Input: part model. Units: mm. Frame: model coordinates. Face numbers are marked on the shaded views. A direction names the side the tool comes from. Give positions to 0.01 mm unless a question says otherwise; leave off trailing zeros. Order: outer loops, then holes, each group sorted by start corner. A loop starts at its lowest first (then second) coordinate and runs counter-clockwise, first axis right, second up. Notation, with made-up numbers: (72, 50.25) - (95, 50.25) arc R11 cw to (95, 68.25) - close; hole circle Ø8 at (-32.75, 61.5). An arc over 180 degrees is marked (long way). Use a Markdown table: item, result.
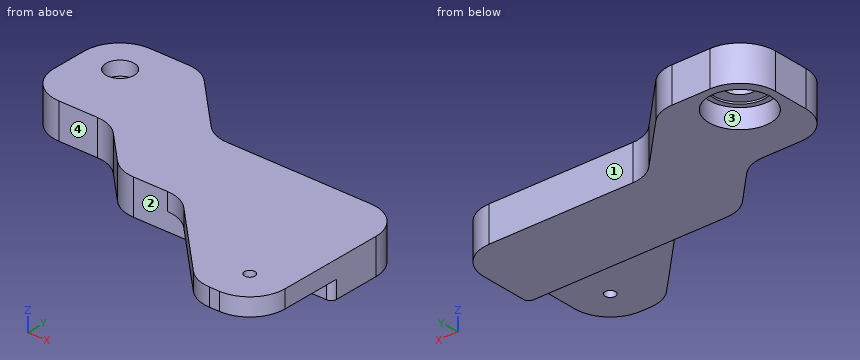
from build123d import *

# Parameters (mm, degrees)
ESQUISSE1_W                  = 200
ESQUISSE1_H                  = 100
BOSS_EXTRU_1_DEPTH           = 20
ENL_V_MAT_EXTRU_1_DEPTH      = 225.499443206
ENL_V_MAT_EXTRU_1_DEPTH_BACK = 225.499443206
ESQUISSE2_R                  = 3
ENL_V_MAT_EXTRU_2_DEPTH      = 225.499443206
ENL_V_MAT_EXTRU_2_DEPTH_BACK = 225.499443206
ENL_V_MAT_EXTRU_3_DEPTH      = 10
ENL_V_MAT_EXTRU_4_DEPTH      = 224.830292856
ENL_V_MAT_EXTRU_4_DEPTH_BACK = 224.830292856
BOSS_EXTRU_2_DEPTH           = 20
ESQUISSE7_R                  = 17.5
ENL_V_MAT_EXTRU_5_DEPTH      = 11
ENL_V_MAT_EXTRU_6_DEPTH      = 245.378804318
ENL_V_MAT_EXTRU_6_DEPTH_BACK = 245.378804318
ESQUISSE8_R                  = 8
ESQUISSE9_R                  = 14.5
ENL_V_MAT_EXTRU_7_DEPTH      = 1
CONG_1_R                     = 20
CONG_2_R                     = 3


with BuildPart() as part:
    # Esquisse1 → Boss.-Extru.1 (new body)
    with BuildSketch(Plane.XY):
        with Locations((100, 50)):
            Rectangle(ESQUISSE1_W, ESQUISSE1_H)
    extrude(amount=BOSS_EXTRU_1_DEPTH)

    # Esquisse2 → Enlèv. mat.-Extru.1 (cut, two sides: drawn at the far end of the back side and taken through both)
    with BuildSketch(Plane.XY.offset(20).offset(-ENL_V_MAT_EXTRU_1_DEPTH_BACK)):
        with Locations((180, 20)):
            Circle(ESQUISSE2_R)
    extrude(amount=ENL_V_MAT_EXTRU_1_DEPTH + ENL_V_MAT_EXTRU_1_DEPTH_BACK, mode=Mode.SUBTRACT)

    # Esquisse3 → Enlèv. mat.-Extru.2 (cut, two sides: drawn at the far end of the back side and taken through both)
    with BuildSketch(Plane.XY.offset(20).offset(-ENL_V_MAT_EXTRU_2_DEPTH_BACK)):
        Polygon((130, 0), (50, 80), (0, 80), (0, 0), align=None)
    extrude(amount=ENL_V_MAT_EXTRU_2_DEPTH + ENL_V_MAT_EXTRU_2_DEPTH_BACK, mode=Mode.SUBTRACT)

    # Esquisse4 → Enlèv. mat.-Extru.3 (cut)
    with BuildSketch(Plane(origin=(0, 0, 0), x_dir=(-1, 0, 0), z_dir=(0, 0, -1))):
        Polygon((-130, 0), (-79, 51), (-200, 51), (-200, 0), align=None)
    extrude(amount=-ENL_V_MAT_EXTRU_3_DEPTH, mode=Mode.SUBTRACT)

    # Esquisse5 → Enlèv. mat.-Extru.4 (cut, two sides: drawn at the far end of the back side and taken through both)
    with BuildSketch(Plane(origin=(0, 0, 10), x_dir=(-1, 0, 0), z_dir=(0, 0, -1)).offset(-ENL_V_MAT_EXTRU_4_DEPTH_BACK)):
        Polygon((-130, 0), (-166, 0), (-115, 51), (-79, 51), align=None)
    extrude(amount=ENL_V_MAT_EXTRU_4_DEPTH + ENL_V_MAT_EXTRU_4_DEPTH_BACK, mode=Mode.SUBTRACT)

    # Esquisse6 → Boss.-Extru.2 (add)
    with BuildSketch(Plane.XY.offset(20)):
        Polygon((0, 100), (90, 100), (50, 140), (0, 140), align=None)
    extrude(amount=-BOSS_EXTRU_2_DEPTH)

    # Esquisse7 → Enlèv. mat.-Extru.5 (cut)
    with BuildSketch(Plane(origin=(0, 0, 0), x_dir=(-1, 0, 0), z_dir=(0, 0, -1))):
        with Locations((-22, 118)):
            Circle(ESQUISSE7_R)
    extrude(amount=-ENL_V_MAT_EXTRU_5_DEPTH, mode=Mode.SUBTRACT)

    # Esquisse8 → Enlèv. mat.-Extru.6 (cut, two sides: drawn at the far end of the back side and taken through both)
    with BuildSketch(Plane(origin=(0, 0, 11), x_dir=(-1, 0, 0), z_dir=(0, 0, -1)).offset(-ENL_V_MAT_EXTRU_6_DEPTH_BACK)):
        with Locations((-22, 118)):
            Circle(ESQUISSE8_R)
    extrude(amount=ENL_V_MAT_EXTRU_6_DEPTH + ENL_V_MAT_EXTRU_6_DEPTH_BACK, mode=Mode.SUBTRACT)

    # Esquisse9 → Enlèv. mat.-Extru.7 (cut)
    with BuildSketch(Plane(origin=(0, 0, 11), x_dir=(-1, 0, 0), z_dir=(0, 0, -1))):
        with Locations((-22, 118)):
            Circle(ESQUISSE9_R)
    extrude(amount=-ENL_V_MAT_EXTRU_7_DEPTH, mode=Mode.SUBTRACT)

    # Congé1
    cong_1_edges = [part.edges().sort_by_distance(p)[0] for p in [
        (0, 80, 10),
        (50, 80, 10),
        (79, 51, 10),
        (115, 51, 15),
        (166, 0, 15),
        (200, 100, 10),
        (0, 140, 10),
        (200, 0, 15),
        (50, 140, 10),
        (90, 100, 10),
    ]]
    fillet(cong_1_edges, radius=CONG_1_R)

    # Congé2
    cong_2_edges = [part.edges().sort_by_distance(p)[0] for p in [
        (200, 51, 5),
    ]]
    fillet(cong_2_edges, radius=CONG_2_R)


solid = part.part
1. Section query A-A (x = 22). Return loops of the section in (y, z), then the cut area to 3 significant figures.
Response:
| item | result |
|---|---|
| outline | (80, 0) - (100.5, 0) - (100.5, 11) - (103.5, 11) - (103.5, 12) - (110, 12) - (110, 20) - (80, 20) - close; (126, 12) - (132.5, 12) - (132.5, 11) - (135.5, 11) - (135.5, 0) - (140, 0) - (140, 20) - (126, 20) - close |
| area | 658 mm^2 |
2. Section query C-C (y = 112). Return loops of the section in (x, z), then the cut area to 3 significant figures.
Response:
| item | result |
|---|---|
| outline | (0, 0) - (5.56, 0) - (5.56, 11) - (8.8, 11) - (8.8, 12) - (16.71, 12) - (16.71, 20) - (0, 20) - close; (27.29, 12) - (35.2, 12) - (35.2, 11) - (38.44, 11) - (38.44, 0) - (78, 0) - (78, 20) - (27.29, 20) - close |
| area | 1,090 mm^2 |
3. Section query B-B (z = 3.25). Return loops of the section in (x, y).
Response:
| item | result |
|---|---|
| outline | (0, 100) arc R20 ccw to (20, 80) - (41.72, 80) arc R20 cw to (55.86, 74.14) - (73.14, 56.86) arc R20 ccw to (87.28, 51) - (197, 51) arc R3 ccw to (200, 54) - (200, 80) arc R20 ccw to (180, 100) - (98.28, 100) arc R20 cw to (84.14, 105.86) - (55.86, 134.14) arc R20 ccw to (41.72, 140) - (20, 140) arc R20 ccw to (0, 120) - close; hole circle Ø35 at (22, 118) |
4. Pin query (flat end, axial travel): pin 1 (12 mm diameter, centred on x = 66.5, z = 17, fed in from +Y); pin 2 (9.5 mm diameter, centred on x = 180, y = 20, fed in from +Z); pin 3 (4 mm diameter, centred on y = 45.5, z = 9.5, fed in from -X); pin 4 (23 mm diameter, centred on x = 22, y = 118, fed in from -Z). Return the tip coordinate at first contact, or that it passes through.
Response:
| item | result |
|---|---|
| pin 1 | stops at y = 129.5 |
| pin 2 | stops at z = 20 |
| pin 3 | stops at x = 118.11 |
| pin 4 | stops at z = 12 |
5. Material intervals for line 1 along Y through (x, z) = (22, 5); line 2 along Y through (x, z) = (22, 11.7); line 3 along Y through (x, z) = (130.5, 7.25), sorted ascending.
Response:
| item | result |
|---|---|
| line 1 | y = 80 to 100.5, 135.5 to 140 |
| line 2 | y = 80 to 103.5, 132.5 to 140 |
| line 3 | y = 51 to 100 |
6. Set-up query: the marked faces 1, 2, 3 and 4. Return all of +Z, -Z, +X, -X, +Y, -Y with unobstructed straight access to the full face (end or side cutting, diameter ignored); none if empty.
Response:
| item | result |
|---|---|
| face 1 | +Z, -Z, +X, +Y |
| face 2 | -Z, -X, -Y |
| face 3 | -Z |
| face 4 | +Z, -Z, -X, -Y |
7. Section query D-D (x = 70.5). Return loops of the section in (y, z).
Response:
| item | result |
|---|---|
| outline | (59.5, 0) - (119.5, 0) - (119.5, 20) - (59.5, 20) - close |
